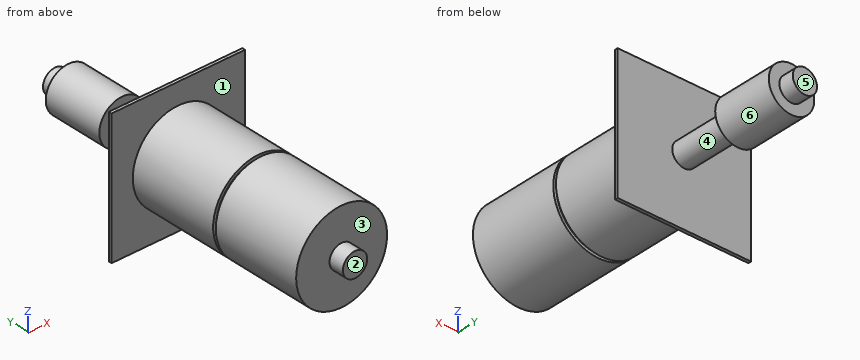
from build123d import *

# Parameters (mm, degrees)
SKETCH1_R           = 15
BOSS_EXTRUDE1_DEPTH = 30
SKETCH2_W           = 44
SKETCH2_H           = 44
BOSS_EXTRUDE2_DEPTH = 1
SKETCH3_R           = 4
BOSS_EXTRUDE3_DEPTH = 20
SKETCH4_R           = 7.5
BOSS_EXTRUDE4_DEPTH = 20
SKETCH5_R           = 4
BOSS_EXTRUDE5_DEPTH = 5
SKETCH6_R           = 14
BOSS_EXTRUDE6_DEPTH = 1
SKETCH7_R           = 15
BOSS_EXTRUDE7_DEPTH = 30
SKETCH8_R           = 4
BOSS_EXTRUDE8_DEPTH = 5


with BuildPart() as part:
    # Sketch1 → Boss-Extrude1 (new body)
    with BuildSketch(Plane(origin=(0, 0, 0), x_dir=(1, 0, 0), z_dir=(0, 1, 0))):
        Circle(SKETCH1_R)
    extrude(amount=BOSS_EXTRUDE1_DEPTH)

    # Sketch2 → Boss-Extrude2 (add)
    with BuildSketch(Plane(origin=(0, 30, 0), x_dir=(1, 0, 0), z_dir=(0, 1, 0))):
        Rectangle(SKETCH2_W, SKETCH2_H)
    extrude(amount=BOSS_EXTRUDE2_DEPTH)

    # Sketch3 → Boss-Extrude3 (add)
    with BuildSketch(Plane(origin=(0, 31, 0), x_dir=(1, 0, 0), z_dir=(0, 1, 0))):
        Circle(SKETCH3_R)
    extrude(amount=BOSS_EXTRUDE3_DEPTH)

    # Sketch4 → Boss-Extrude4 (add)
    with BuildSketch(Plane(origin=(0, 51, 0), x_dir=(1, 0, 0), z_dir=(0, 1, 0))):
        Circle(SKETCH4_R)
    extrude(amount=BOSS_EXTRUDE4_DEPTH)

    # Sketch5 → Boss-Extrude5 (add)
    with BuildSketch(Plane(origin=(0, 71, 0), x_dir=(1, 0, 0), z_dir=(0, 1, 0))):
        Circle(SKETCH5_R)
    extrude(amount=BOSS_EXTRUDE5_DEPTH)

    # Sketch6 → Boss-Extrude6 (add)
    with BuildSketch(Plane(origin=(0, 0, 0), x_dir=(-1, 0, 0), z_dir=(0, -1, 0))):
        Circle(SKETCH6_R)
    extrude(amount=BOSS_EXTRUDE6_DEPTH)

    # Sketch7 → Boss-Extrude7 (add)
    with BuildSketch(Plane(origin=(0, -1, 0), x_dir=(-1, 0, 0), z_dir=(0, -1, 0))):
        Circle(SKETCH7_R)
    extrude(amount=BOSS_EXTRUDE7_DEPTH)

    # Sketch8 → Boss-Extrude8 (add)
    with BuildSketch(Plane(origin=(0, -31, 0), x_dir=(-1, 0, 0), z_dir=(0, -1, 0))):
        Circle(SKETCH8_R)
    extrude(amount=BOSS_EXTRUDE8_DEPTH)


solid = part.part
Source: CAD feature listing. Evaluate the final solid. Frame: model axes, mm. Face numbers are marked on the shaded views. A direction names the side the tool comes from. Give positions to 0.01 mm unless a question says otherwise; leave off trailing zeros. Write each loop counter-clockwise with the first axis right and the second up, starting at its lowest first coordinate (ties: lowest second). Pieces come first, ordered by that corner, then holes. Notation, with made-up numbers: (85, 48.5) -> (91, 48.5) arc R28 cw to (91, 76.5) -> close; hole circle Ø1 at (82.5, -34.5). An arc over 180 degrees is marked (long way). Return JSON: item names as keys, results as strings. Group by question number.
1. Section C-C, the plane y = 43.5. Output: boundary loops of the cut face in (x, z).
2. Mould query, pull axis Y, two halves, no side actions, for the marked faces 3, 4, 5 and 6. Classes: +Y half, -Y half, draft (parallel to the pull), parting line (faces both ways), or undercut.
3. Section D-D, the plane x = -9. Output: boundary loops of the cut face in (y, z), then the cut area to 3 significant figures.
4. Access query for the marked faces 1 and 2. Directions: +Z, -Z, +X, -X, +Y, -Y. A direction counts if a zero-diameter tool reaches every point of the face in a straight line with its end or side. Return the directions, or none.
5. Pin query (flat end, axial travel): pin 1 Ø10 at (x, y) = (-5.5, 22) entering from -Z; pin 2 Ø1.5 at (x, y) = (-11.5, 8.5) entering from +Z; pin 3 Ø2 at (y, z) = (-9.5, -13.5) entering from -X. Return the tip coordinate at first contact, or that it passes through.
6. Material intervals for line 1 (Y direction, x = 7, z = -14); line 2 (X direction, y = 7.5, z = 10.5); line 3 (X direction, y = -6, z = -7.5), sorted ascending. Write a range as from..to.
Determined:
{
 "1": {"outline": "circle Ø8 at (0, 0)"},
 "2": {"face 3": "-Y half", "face 4": "undercut", "face 5": "+Y half", "face 6": "draft"},
 "3": {"outline": "(-31, -12) -> (-1, -12) -> (-1, -10.72) -> (0, -10.72) -> (0, -12) -> (30, -12) -> (30, -22) -> (31, -22) -> (31, 22) -> (30, 22) -> (30, 12) -> (0, 12) -> (0, 10.72) -> (-1, 10.72) -> (-1, 12) -> (-31, 12) -> close", "area": "1,510 mm2"},
 "4": {"face 1": "-Y", "face 2": "+Z, -Z, +X, -X, -Y"},
 "5": {"pin 1": "stops at z = -14.99", "pin 2": "stops at z = 10.46", "pin 3": "stops at x = -8.29"},
 "6": {"line 1": "y = 30..31", "line 2": "x = -10.71..10.71", "line 3": "x = -12.99..12.99"}
}
